```python
from build123d import *

# Parameters (mm, degrees)
SKETCH1_R           = 1.875
BOSS_EXTRUDE1_DEPTH = 3
FILLET1_R           = 2
SKETCH2_R           = 3.75
BOSS_EXTRUDE2_DEPTH = 4


with BuildPart() as part:
    # Sketch1 → Boss-Extrude1 (new body)
    with BuildSketch(Plane.XY):
        with BuildLine():
            Line((-20.997727651, -1.013441276), (-30.997581376, -1.013441276))
            ThreePointArc((-30.997581376, -1.013441276), (-32.411794939, -1.599227714), (-32.997581376, -3.013441276))
            Line((-32.997581376, -3.013441276), (-32.997581376, -57.013441276))
            ThreePointArc((-32.997581376, -57.013441276), (-32.411794939, -58.427654839), (-30.997581376, -59.013441276))
            Line((-30.997581376, -59.013441276), (-20.997727651, -59.013441276))
            ThreePointArc((-20.997727651, -59.013441276), (-19.583514088, -58.427654839), (-18.997727651, -57.013441276))
            Line((-18.997727651, -57.013441276), (-18.997727651, -41.251974862))
            ThreePointArc((-18.997727651, -41.251974862), (-19.354888824, -40.111325665), (-20.298808241, -39.378072073))
            ThreePointArc((-20.298808241, -39.378072073), (-26.804211193, -30.008558133), (-20.298808241, -20.639044193))
            ThreePointArc((-20.298808241, -20.639044193), (-19.354888824, -19.905790602), (-18.997727651, -18.765141405))
            Line((-18.997727651, -18.765141405), (-18.997727651, -3.013441276))
            ThreePointArc((-18.997727651, -3.013441276), (-19.583514088, -1.599227714), (-20.997727651, -1.013441276))
        make_face()
        with Locations((-26.501848256, -15.008558747)):
            Circle(SKETCH1_R, mode=Mode.SUBTRACT)
        with Locations((-26.501848256, -45.008558747)):
            Circle(SKETCH1_R, mode=Mode.SUBTRACT)
    extrude(amount=BOSS_EXTRUDE1_DEPTH)

    # Fillet1
    fillet1_edges = [part.edges().sort_by_distance(p)[0] for p in [
        (-19.354888824, -40.111325665, 3),
        (-26.804211193, -30.008558133, 3),
        (-19.354888824, -19.905790602, 3),
        (-18.997727651, -10.889291341, 3),
        (-19.583514088, -1.599227714, 3),
        (-25.997654514, -1.013441276, 3),
        (-32.411794939, -1.599227714, 3),
        (-32.997581376, -30.013441276, 3),
        (-32.411794939, -58.427654839, 3),
        (-25.997654514, -59.013441276, 3),
        (-19.583514088, -58.427654839, 3),
        (-18.997727651, -49.132708069, 3),
    ]]
    fillet(fillet1_edges, radius=FILLET1_R)

    # Sketch2 → Boss-Extrude2 (add)
    with BuildSketch(Plane.XY.offset(3)):
        with Locations((-26.501848256, -7.508558747)):
            Circle(SKETCH2_R)
        with Locations((-26.501848256, -52.508558747)):
            Circle(SKETCH2_R)
    extrude(amount=-BOSS_EXTRUDE2_DEPTH)


solid = part.part
```
Part model, mm, in its own coordinate system. A direction names the side the tool comes from. Coordinates: 2 decimals unless noted, no trailing zeros. Order: outer loops, then holes, each group sorted by start corner. A loop starts at its lowest first (then second) coordinate and runs counter-clockwise, first axis right, second up. Notation, with made-up numbers: (5.5, 73.25) - (37.5, 73.25) arc R15 cw to (37.5, 92.25) - close; hole circle Ø4 at (60, -37.5). An arc over 180 degrees is marked (long way). Return JSON: item names as keys, results as strings. Group by question number.
Item 1: Pull direction Y, two halves, no side cores. Call faces 4 (the face through (-32.43, -58.41, 0.49)), 5 (the face through (-23.038, -8.945, -0.493)), 6 (the face through (-32.998, -29.6, 0.5)), 7 (the face through (-25.9, -1.013, 0.5)): pulls with the +Y half, pulls with the -Y half, needs draft (parallel to the pull), parting line crosses it, or undercut.
Item 2: Cut at B-B (z = -0.5). List the corners of the cut face in (x, y).
Item 3: Cut at C-C (y = -51). List the corners of the cut face in (x, z), plus the area to 3 significant figures.
Item 4: Cut at A-A (z = 1.7). State how many separate pieces and enclosed holes the cut face has, plus the area to 3 significant figures.
Item 5: Which spindle directions (+Z, -Z, +X, -X, +Y, -Y) get a long thin tool onto all of the face, cutting with end or side? Do faces 1 (the face through (-19.345, -40.125, 0.493)), 2 (the face through (-19.568, -1.615, 0.493)), 3 (the face through (-24.771, -55.835, -0.493)). Say none if no direction does.
Item 6: Drill centre lines: probe 1 along X at (y, z) = (-15, 1); probe 2 along Z at (x, y) = (-30.5, -9.5); probe 3 along X at (y, z) = (-16, 1.25). Where is each one in solid material? Low to high. Write a range as from..to.
Item 7: Pin check, flat tips, straight feed: pin 1 (8 mm diameter, centred on x = -21.5, y = -22.5, fed in from -Z); pin 2 (1 mm diameter, centred on x = -23.5, z = 1.5, fed in from -Y); pin 3 (4 mm diameter, centred on x = -24.5, y = -25.5, fed in from +Z). Stop position of each tip, or through.
Check values:
{
 "1": {"face 4": "pulls with the -Y half", "face 5": "undercut", "face 6": "needs draft", "face 7": "pulls with the +Y half"},
 "2": {"outline": "circle Ø7.5 at (-26.5, -52.51); circle Ø7.5 at (-26.5, -7.51)"},
 "3": {"outline": "(-33, 0) - (-29.94, 0) - (-29.94, -1) - (-23.07, -1) - (-23.07, 0) - (-19, 0) - (-19, 1) arc R2 ccw to (-21, 3) - (-31, 3) arc R2 ccw to (-33, 1) - close", "area": "47.1 mm2"},
 "4": {"separate pieces": "1", "enclosed holes": "2", "area": "654 mm2"},
 "5": {"face 1": "+Z, -Z, +X", "face 2": "+Z, -Z, +X, +Y", "face 3": "-Z"},
 "6": {"probe 1": "x = -33..-28.38, -24.63..-19", "probe 2": "z = 0..3", "probe 3": "x = -32.98..-28.09, -24.91..-19.01"},
 "7": {"pin 1": "stops at z = 0", "pin 2": "stops at y = -59.01", "pin 3": "stops at z = 2.68"}
}
